Can you work these out from the model? Positions are in its coordinate system, mm. A direction names the side the tool comes from. Give positions to 0.01 mm unless a question says otherwise; leave off trailing zeros. Loops run counter-clockwise (first coordinate to the right, second up) from the corner with the lowest first, then second, coordinate; pieces in that order, holes last.
from build123d import *

# Parameters (mm, degrees)
ESTRUSIONE1_DEPTH                                    = 200
M10_LAMATURA_PER_VITE_A_COPERTURA_CILIND_D           = 11
M10_LAMATURA_PER_VITE_A_COPERTURA_CILIND_CBORE_D     = 18
M10_LAMATURA_PER_VITE_A_COPERTURA_CILIND_CBORE_DEPTH = 10
RIPETIZIONE_A_L1_COUNT                               = 5
RIPETIZIONE_A_L1_PITCH                               = 42
RIPETIZIONE_A_L1_COUNT_DIR2                          = 2
RIPETIZIONE_A_L1_PITCH_DIR2                          = 160
SMUSSO1_SIZE                                         = 3
SMUSSO2_SIZE                                         = 2


with BuildPart() as part:
    # Schizzo1 → Estrusione1 (new body)
    with BuildSketch(Plane(origin=(0, 0, 0), x_dir=(1, 0, 0), z_dir=(0, 1, 0))):
        Polygon((0, -95), (0, 95), (30, 95), (30, 90), (25, 90), (25, 70), (30, 70), (30, 66), (30, 26.5), (16, 21.5), (16, -21.5), (30, -26.5), (30, -66), (30, -70), (25, -70), (25, -90), (30, -90), (30, -95), align=None)
    extrude(amount=ESTRUSIONE1_DEPTH)

    # M10 Lamatura per vite a copertura cilindrica esagonale1 (through all)
    with Locations(Plane.ZY):
        with Locations((80, 184)):
            m10_lamatura_per_vite_a_copertura_cilind = CounterBoreHole(M10_LAMATURA_PER_VITE_A_COPERTURA_CILIND_D / 2, M10_LAMATURA_PER_VITE_A_COPERTURA_CILIND_CBORE_D / 2, M10_LAMATURA_PER_VITE_A_COPERTURA_CILIND_CBORE_DEPTH)

    # Ripetizione a L1: M10 Lamatura per vite a copertura cilind 5 × 2
    with Locations(*[(0, -i * RIPETIZIONE_A_L1_PITCH, -j * RIPETIZIONE_A_L1_PITCH_DIR2) for i in range(RIPETIZIONE_A_L1_COUNT) for j in range(RIPETIZIONE_A_L1_COUNT_DIR2) if (i, j) != (0, 0)]):
        add(m10_lamatura_per_vite_a_copertura_cilind, mode=Mode.SUBTRACT)

    # Smusso1
    smusso1_edges = [part.edges().sort_by_distance(p)[0] for p in [
        (0, 100, 95),
        (0, 100, -95),
    ]]
    chamfer(smusso1_edges, length=SMUSSO1_SIZE)

    # Smusso2
    smusso2_edges = [part.edges().sort_by_distance(p)[0] for p in [
        (30, 200, 48.25),
        (23, 200, 24),
        (16, 200, 0),
        (23, 200, -24),
        (30, 200, -48.25),
    ]]
    chamfer(smusso2_edges, length=SMUSSO2_SIZE)


solid = part.part
(1) Will these pins go through, and if not, where does the flat tip stop? P1, Ø14.5, axis at y = 58, z = 80, coming from the +X side; P2, Ø14.5, axis at y = 100, z = 80, coming from the -X side.
Returned:
P1: stops at x = 25
P2: stops at x = 10
(2) Thinking about a two-plate mould opening in Z: for faces 1 (the flat face through (27, 99, 90)), 2 (the flat face through (17, 99, 95)), 3 (the flat face through (30, 98, -48)), which applies, pulls with the +Z half, pulls with the -Z half, needs draft (parallel to the pull), parting line crosses it, or undercut?
Returned:
face 1: undercut
face 2: pulls with the +Z half
face 3: needs draft
(3) Suppose I cut it at A-A on x = 18.5. Give the number of separate pieces and of enclosed holes in the cut face, plus the area to 3 significant figures.
Returned:
separate pieces: 2
enclosed holes: 10
area: 28,100 mm2
(4) Which directions (+Z, -Z, +X, -X, +Y, -Y) give clear straight access to the entire face, cutting with the end or side of a thin tool? Please do faces 4 (the cylindrical face through (4.93, 191.59, -75.16)), 5 (the flat face through (22.112, 198.986, -24.73)), 6 (the flat face through (28, 99, -90)).
Returned:
face 4: -X
face 5: +X, +Y
face 6: +X, +Y, -Y
(5) Suppose I cut it at B-B on y = 163. List the corners of the cut face in (x, z) for me.
Returned:
outline: (0, -92) - (3, -95) - (30, -95) - (30, -90) - (25, -90) - (25, -70) - (30, -70) - (30, -26.5) - (16, -21.5) - (16, 21.5) - (30, 26.5) - (30, 70) - (25, 70) - (25, 90) - (30, 90) - (30, 95) - (3, 95) - (0, 92) - close
(6) Please list where these lines run through material, in increasing order: probe 1 along Y at (x, z) = (4.75, -80); probe 2 along Z at (x, y) = (18.25, 12); probe 3 along Z at (x, y) = (28.75, 96.5).
Returned:
probe 1: y = 0 to 7, 25 to 49, 67 to 91, 109 to 133, 151 to 175, 193 to 200
probe 2: z = -95 to -83.77, -76.23 to -22.3, 22.3 to 76.23, 83.77 to 95
probe 3: z = -95 to -90, -70 to -26.05, 26.05 to 70, 90 to 95
